```python
from build123d import *

# Parameters (mm, degrees)
CROQUIS1_R              = 100
SALIENTE_EXTRUIR1_DEPTH = 3
CROQUIS3_R              = 110
CORTAR_EXTRUIR1_DEPTH   = 3
REDONDEO1_R             = 10
CORTAR_EXTRUIR2_DEPTH   = 142.453172607
CROQUIS5_R              = 1.5
CORTAR_EXTRUIR3_DEPTH   = 10


with BuildPart() as part:
    # Croquis1 → Saliente-Extruir1 (new body)
    with BuildSketch(Plane.XY):
        Circle(CROQUIS1_R)
    extrude(amount=SALIENTE_EXTRUIR1_DEPTH)

    # Croquis3 → Cortar-Extruir1 (cut)
    with BuildSketch(Plane.XY.offset(3)):
        with Locations((190, 0)):
            Circle(CROQUIS3_R)
    extrude(amount=-CORTAR_EXTRUIR1_DEPTH, mode=Mode.SUBTRACT)

    # Redondeo1
    redondeo1_edges = [part.edges().sort_by_distance(p)[0] for p in [
        (89.473684211, -44.659375654, 1.5),
        (89.473684211, 44.659375654, 1.5),
    ]]
    fillet(redondeo1_edges, radius=REDONDEO1_R)

    # Croquis4 → Cortar-Extruir2 (cut, through all)
    with BuildSketch(Plane.XY.offset(3)):
        Polygon((-83.792153571, -57.629202667), (-57.629202667, -83.792153571), (-42.072853481, -68.235804385), (-45.290189335, -65.01846853), (-8.520636713, -28.248915908), (-28.248915908, -8.520636713), (-65.01846853, -45.290189335), (-68.235804385, -42.072853481), align=None)
        Polygon((-8.520636713, 31.077343033), (-28.248915908, 11.349063838), (-65.01846853, 48.11861646), (-68.235804385, 44.901280605), (-83.792153571, 60.457629791), (-57.629202667, 86.620580695), (-42.072853481, 71.064231509), (-45.290189335, 67.846895655), align=None)
        Polygon((31.077343033, 11.349063838), (11.349063838, 31.077343033), (48.11861646, 67.846895655), (44.901280605, 71.064231509), (60.457629791, 86.620580695), (86.620580695, 60.457629791), (71.064231509, 44.901280605), (67.846895655, 48.11861646), align=None)
        Polygon((11.349063838, -28.248915908), (31.077343033, -8.520636713), (67.846895655, -45.290189335), (71.064231509, -42.072853481), (86.620580695, -57.629202667), (60.457629791, -83.792153571), (44.901280605, -68.235804385), (48.11861646, -65.01846853), align=None)
    extrude(amount=-CORTAR_EXTRUIR2_DEPTH, mode=Mode.SUBTRACT)

    # Croquis5 → Cortar-Extruir3 (cut)
    with BuildSketch(Plane.XY.offset(3)):
        with Locations((-64.311361749, -40.340441867)):
            Circle(CROQUIS5_R)
        with Locations((-48.401459172, -24.43053929)):
            Circle(CROQUIS5_R)
        with Locations((-24.43053929, -48.401459172)):
            Circle(CROQUIS5_R)
        with Locations((-40.340441867, -64.311361749)):
            Circle(CROQUIS5_R)
        with Locations((-24.43053929, 51.229886297)):
            Circle(CROQUIS5_R)
        with Locations((-40.340441867, 67.139788874)):
            Circle(CROQUIS5_R)
        with Locations((-48.401459172, 27.258966415)):
            Circle(CROQUIS5_R)
        with Locations((-64.311361749, 43.168868991)):
            Circle(CROQUIS5_R)
        with Locations((51.229886297, 27.258966415)):
            Circle(CROQUIS5_R)
        with Locations((67.139788874, 43.168868991)):
            Circle(CROQUIS5_R)
        with Locations((27.258966415, 51.229886297)):
            Circle(CROQUIS5_R)
        with Locations((43.168868991, 67.139788874)):
            Circle(CROQUIS5_R)
        with Locations((27.258966415, -48.401459172)):
            Circle(CROQUIS5_R)
        with Locations((43.168868991, -64.311361749)):
            Circle(CROQUIS5_R)
        with Locations((51.229886297, -24.43053929)):
            Circle(CROQUIS5_R)
        with Locations((67.139788874, -40.340441867)):
            Circle(CROQUIS5_R)
    extrude(amount=-CORTAR_EXTRUIR3_DEPTH, mode=Mode.SUBTRACT)


solid = part.part
```
Part model, mm, in its own coordinate system. A direction names the side the tool comes from. Coordinates: 2 decimals unless noted, no trailing zeros. Loops run counter-clockwise (first coordinate to the right, second up) from the corner with the lowest first, then second, coordinate; pieces in that order, holes last. Notation, with made-up numbers: (65, -13) - (81, -13) arc R37 ccw to (81, 23) - close; hole circle Ø7 at (67, 52). An arc over 180 degrees is marked (long way). Write item = value, one per line. Start each with the question number.
Item 1: Cut at D-D, the plane z = 1.65. State how many separate pieces and enclosed holes the cut face has, and give its area (3 significant figures).
Item 2: Cut at C-C, the plane y = 8.5. Give the cut face in (x, z).
Item 3: Cut at A-A, the plane x = 39. Give the cut face in (y, z).
Item 4: Mould opens along X. For faces 5 (the flat face through (-46.38, -26.65, 1.52)), 6 (the cylindrical face through (-99.983, 1.869, 1.479)), 7 (the flat face through (-7, 1, 3)) say: released by +X, released by -X, zero draft, split by the parting line, or undercut.
Item 5: Flat gauge pins, fed straight in: pin 1 Ø1.5 at (y, z) = (-33.5, 0.5) entering from +X; pin 2 Ø1.5 at (y, z) = (-1.5, 1) entering from -X; pin 3 Ø2.5 at (x, y) = (-64.31, -40.34) entering from -Z; pin 4 Ø1.5 at (x, z) = (-35.5, 2) entering from -Y. Where does each tip first touch, or does it go through?
Item 6: 3-axis set-ups, long thin cutter, end or side, ignore diameter. For faces 1 (the flat face through (-75.303, -49.14, 1.521)), 2 (the flat face through (-18.2, 21.4, 1.5)), 3 (the flat face through (51.58, -74.914, 1.521)), 4 (the flat face through (-49.341, -75.504, 1.521)): which of +Z, -Z, +X, -X, +Y, -Y reach the whole face in a straight line?
Item 7: Wall check: L1, parallel to X at y = -64, z = 0.5; L2, parallel to X at y = 38.5, z = 1.5; L3, parallel to Y at x = -25, z = 0.2. Give the ranges that are in metal, low to high. Write a range as from..to.
Item 8: Cut at B-B, the plane y = -13. Give the cut face in (x, z), and give its area (3 significant figures).
The answers:
q1.separate_pieces = 1
q1.enclosed_holes = 16
q1.area = 21,400 mm2
q2.outline = (-99.64, 0) - (80.33, 0) - (80.33, 3) - (-99.64, 3) - close
q3.outline = (-92.08, 0) - (-55.9, 0) - (-55.9, 3) - (-92.08, 3) - close; (-16.44, 0) - (19.27, 0) - (19.27, 3) - (-16.44, 3) - close; (58.73, 0) - (92.08, 0) - (92.08, 3) - (58.73, 3) - close
q4.face_5 = undercut
q4.face_6 = released by -X
q4.face_7 = zero draft
q5.pin_1 = 85.47
q5.pin_2 = -100
q5.pin_3 = through
q5.pin_4 = -93.77
q6.face_1 = +Z, -Z, -Y
q6.face_2 = +Z, -Z
q6.face_3 = +Z, -Z, +X
q6.face_4 = +Z, -Z, -X
q7.L1 = -44.27..-41.81, -38.87..41.7, 44.64..47.1
q7.L2 = -92.29..-55.4, -15.94..18.77, 58.23..86.96
q7.L3 = -96.82..-49.79, -47.01..-44.73, -11.77..14.6, 47.56..49.84, 52.62..96.82
q8.outline = (-99.15, 0) - (-32.73, 0) - (-32.73, 3) - (-99.15, 3) - close; (-23.77, 0) - (26.6, 0) - (26.6, 3) - (-23.77, 3) - close; (35.56, 0) - (80.77, 0) - (80.77, 3) - (35.56, 3) - close
q8.area = 486 mm2
